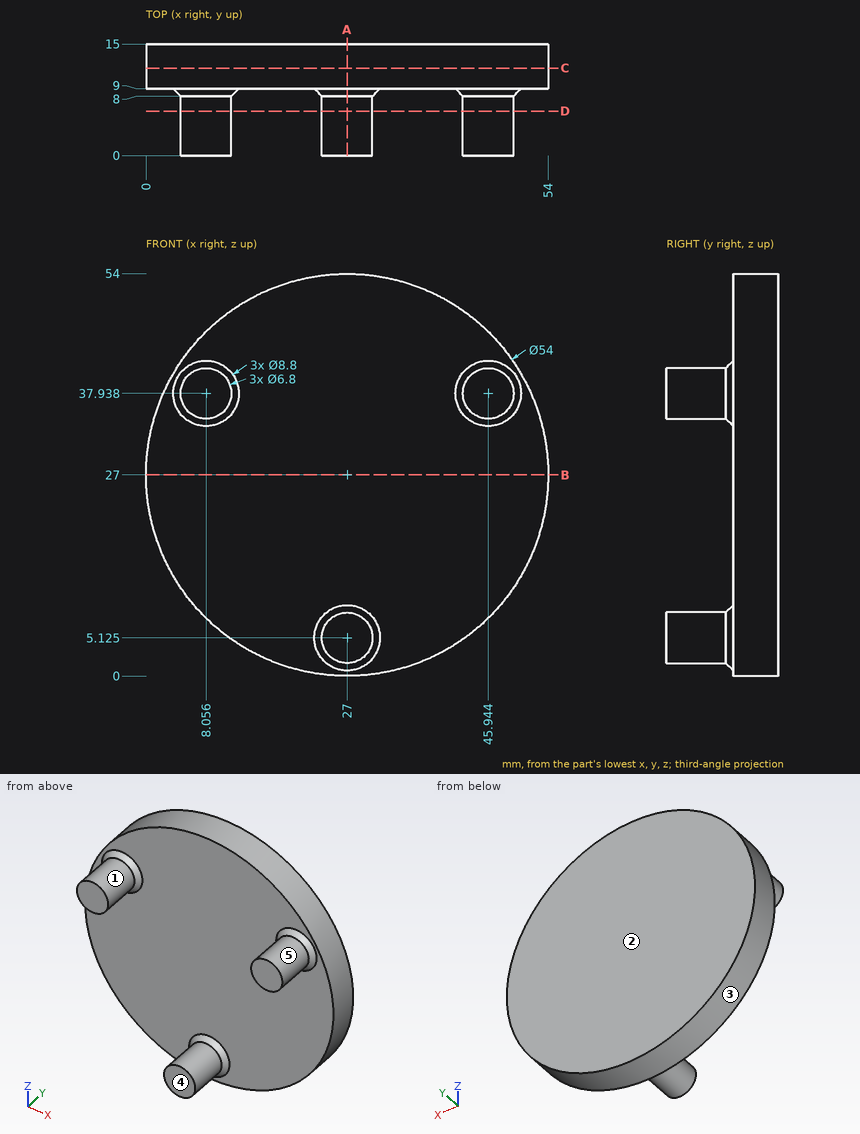
For this review, use the dimensioned drawing (mm, ordinates from the lowest corner) and the shaded views. A direction names the side the tool comes from. Coordinates: 2 decimals unless noted, no trailing zeros. Write each loop counter-clockwise with the first axis right and the second up, starting at its lowest first coordinate (ties: lowest second). Pieces come first, ordered by that corner, then holes. Notation, with made-up numbers: (46.25, 89) - (68.25, 89) arc R20 cw to (68.25, 117) - close; hole circle Ø10 at (-18.75, 38.5). An arc over 180 degrees is marked (long way). Answer in a Markdown table with one row per item. Add a question column.
Q1. Consider section C-C on y = 11.75. Give the boundary of the cut face in (x, z).
Q2. Consider section B-B on z = 27. Give the boundary of the cut face in (x, y).
Q3. Draft analysis for pull direction X (two halves, no side actions). For the marked faces 3, 4 and 5, state which applies: +X half, -X half, draft (parallel to the pull), parting line (faces both ways), or undercut.
Q4. Consider section A-A on x = 27. Give the boundary of the cut face in (y, z) (1 decimal).
Q5. Consider section D-D on y = 6. Give the boundary of the cut face in (x, z) (1 decimal).
Q6. For the marked faces 1 and 2, list the 3-axis set-ups (+Z, -Z, +X, -X, +Y, -Y) from which the entire face can be reached by the end or side of a thin tool; tool diameter is ignored.
Q7. Clearance check with flat-ended pins moving along their axes: pin 1 (5 mm diameter, centred on y = 12, z = 43.5, fed in from +X); pin 2 (16 mm diameter, centred on x = 29.5, z = 30.5, fed in from -Y); pin 3 (3 mm diameter, centred on x = 19, y = 11.5, fed in from -Z); pin 4 (3 mm diameter, centred on x = 27, y = 8.5, fed in from +Z). State where each tip first meets the part, or that it passes through.
Q8. To check wall thickness, follow line 1 along Y through (x, z) = (10.5, 44.5); line 2 along X through (y, z) = (3, 41) (1 decimal); line 3 along Z through (x, y) = (26, 14.25). State the ranges of each line that lie inside material, in increasing order. Write a range as from..to.
Answers below:
| question | item | result |
|---|---|---|
| 1 | outline | circle Ø54 at (27, 27) |
| 2 | outline | (0, 9) - (54, 9) - (54, 15) - (0, 15) - close |
| 3 | face 3 | parting line |
| 3 | face 4 | draft |
| 3 | face 5 | undercut |
| 4 | outline | (0, 1.7) - (8, 1.7) - (9, 0.7) - (9, 0) - (15, 0) - (15, 54) - (9, 54) - (9, 9.5) - (8, 8.5) - (0, 8.5) - close |
| 5 | outline | circle Ø6.8 at (8.1, 37.9); circle Ø6.8 at (27, 5.1); circle Ø6.8 at (45.9, 37.9) |
| 6 | face 1 | -Y |
| 6 | face 2 | +Z, -Z, +X, -X, +Y |
| 7 | pin 1 | x = 50.09 |
| 7 | pin 2 | y = 9 |
| 7 | pin 3 | z = 0.79 |
| 7 | pin 4 | z = 54 |
| 8 | line 1 | 9..15 |
| 8 | line 2 | 6.6..9.5, 44.5..47.4 |
| 8 | line 3 | 0.02..53.98 |
